```python
from build123d import *

# Parameters (mm, degrees)
CHAMFER1_SIZE      = 1
SKETCH5_R          = 3
CUT_EXTRUDE1_DEPTH = 60
SKETCH7_R          = 2.5
CUT_EXTRUDE2_DEPTH = 25


with BuildPart() as part:
    # Sketch3 → Revolve1 (revolve)
    with BuildSketch(Plane(origin=(0, 0, 0), x_dir=(1, 0, 0), z_dir=(0, 1, 0))):
        with BuildLine():
            Line((-33, 9.5), (33, 9.5))
            Line((33, 9.5), (33, 6.5))
            Line((33, 6.5), (49, 6.5))
            Line((49, 6.5), (49, 0))
            Line((49, 0), (-48, 0))
            Line((-48, 0), (-48, 3))
            Line((-48, 3), (-48.375, 3))
            ThreePointArc((-48.375, 3), (-48.816941738, 3.183058262), (-49, 3.625))
            Line((-49, 3.625), (-49, 5.5))
            ThreePointArc((-49, 5.5), (-48.707106781, 6.207106781), (-48, 6.5))
            Line((-48, 6.5), (-33, 6.5))
            Line((-33, 6.5), (-33, 9.5))
        make_face()
    revolve(axis=Axis((49, 0, 0), (-1, 0, 0)))

    # Chamfer1
    chamfer1_edges = [part.edges().sort_by_distance(p)[0] for p in [
        (49, 0, 6.5),
    ]]
    chamfer(chamfer1_edges, length=CHAMFER1_SIZE)

    # Sketch5 → Cut-Extrude1 (cut)
    with BuildSketch(Plane.ZY.offset(48)):
        with Locations(Location((0, 0, 0), (0, 0, 180))):
            Circle(SKETCH5_R)
    extrude(amount=-CUT_EXTRUDE1_DEPTH, mode=Mode.SUBTRACT)

    # Sketch7 → Cut-Extrude2 (cut, symmetric)
    with BuildSketch(Plane.XY):
        Circle(SKETCH7_R)
    extrude(amount=CUT_EXTRUDE2_DEPTH, both=True, mode=Mode.SUBTRACT)


solid = part.part
```
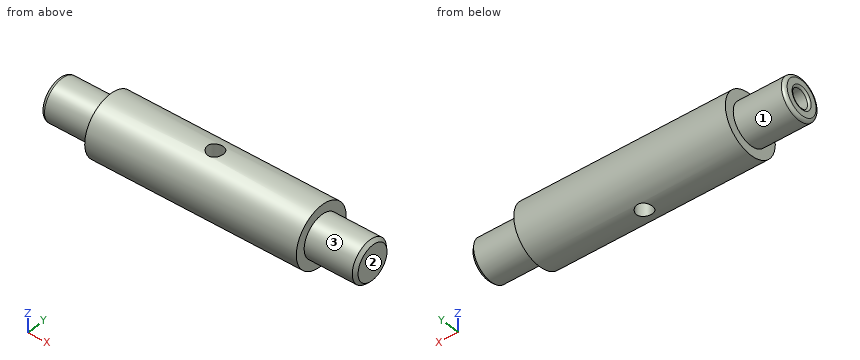
Check sheet for the modelled part. Datum: model origin and axes. Units: mm. Face numbers are marked on the shaded views. A direction names the side the tool comes from. Round coordinates to 2 decimals unless told otherwise and drop trailing zeros. Order: outer loops, then holes, each group sorted by start corner. A loop starts at its lowest first (then second) coordinate and runs counter-clockwise, first axis right, second up.
1) Tool access check on the marked faces 1, 2 and 3. Record the directions out of +Z, -Z, +X, -X, +Y, -Y that give a thin tool (end or side, any length) a straight path to the whole face; none if there is none.
2) Go/stop test with flat-tipped pins: pin 1 Ø4 at (x, z) = (24, -4.5) entering from -Y; pin 2 Ø1.5 at (y, z) = (-6.5, -1.5) entering from -X; pin 3 Ø3 at (x, y) = (26, 5.5) entering from -Z; pin 4 Ø4.5 at (x, y) = (0, 0) entering from -Z. Record where each tip stops, or that it passes through.
3) Scan lines: line 1 (Z direction, x = -34.5, y = 0); line 2 (Z direction, x = -18.5, y = 0); line 3 (X direction, y = 0, z = -5.5). Record each from-to range of solid material in increasing order.
4) Section check B-B (x = 0). Record the boundary of the cut face in (y, z).
5) Section check D-D (x = 36). Record the boundary of the cut face in (y, z), and give its area (3 significant figures).
6) Section check A-A (y = 0). Give the number of separate pieces and of enclosed holes in the cut face, and give its area (3 significant figures).
7) Section check C-C (z = 0). Record the boundary of the cut face in (x, y) (3 decimals).
Result:
1. face 1: -X
1. face 2: +Z, -Z, +X, +Y, -Y
1. face 3: +X
2. pin 1: stops at y = -9.17
2. pin 2: stops at x = -48.91
2. pin 3: stops at z = -8.62
2. pin 4: passes through
3. line 1: z = -6.5 to -3, 3 to 6.5
3. line 2: z = -9.5 to -3, 3 to 9.5
3. line 3: x = -49 to -2.5, 2.5 to 49
4. outline: (-2.5, -9.17) - (-2.5, -1.66) arc R3 cw to (-2.5, 1.66) - (-2.5, 9.17) arc R9.5 ccw to start; (2.5, -9.17) arc R9.5 ccw to (2.5, 9.17) - (2.5, 1.66) arc R3 cw to (2.5, -1.66) - close
5. outline: circle Ø13 at (0, 0)
5. area: 133 mm2
6. separate pieces: 3
6. enclosed holes: 0
6. area: 1,240 mm2
7. outline: (-49, -5.5) arc R1 ccw to (-48, -6.5) - (-33, -6.5) - (-33, -9.5) - (33, -9.5) - (33, -6.5) - (48, -6.5) - (49, -5.5) - (49, 5.5) - (48, 6.5) - (33, 6.5) - (33, 9.5) - (-33, 9.5) - (-33, 6.5) - (-48, 6.5) arc R1 ccw to (-49, 5.5) - (-49, 3.625) arc R0.625 ccw to (-48.375, 3) - (12, 3) - (12, -3) - (-48.375, -3) arc R0.625 ccw to (-49, -3.625) - close
